The listing builds one solid part. Answer for the finished solid, in the listing's coordinates (mm). A direction names the side the tool comes from. Give positions to 0.01 mm unless a question says otherwise; leave off trailing zeros. Order: outer loops, then holes, each group sorted by start corner. A loop starts at its lowest first (then second) coordinate and runs counter-clockwise, first axis right, second up. Notation, with made-up numbers: (73, 29) - (96, 29) arc R25 cw to (96, 60) - close; hole circle Ø10 at (56, -4). An arc over 180 degrees is marked (long way). Answer in a Markdown table with one row per item.
from build123d import *

# Parameters (mm, degrees)
EXTRUDE1_DEPTH = 3.175
EXTRUDE2_DEPTH = 2.8575


with BuildPart() as part:
    # Sketch1 → Extrude1 (new body)
    with BuildSketch(Plane(origin=(0, 0, 0), x_dir=(1, 0, 0), z_dir=(0, 1, 0))):
        with BuildLine():
            Line((3.175, 44.50785877), (45.047498502, 44.50785877))
            ThreePointArc((45.047498502, 44.50785877), (46.651643951, 44.072811758), (47.81618078, 42.886893339))
            Line((47.81618078, 42.886893339), (87.038547596, -26.992036046))
            ThreePointArc((87.038547596, -26.992036046), (87.009818306, -30.150216064), (84.269865318, -31.721070615))
            Line((84.269865318, -31.721070615), (32.528914715, -31.721070615))
            ThreePointArc((32.528914715, -31.721070615), (30.778624678, -31.195053398), (29.608292243, -29.791297251))
            Line((29.608292243, -29.791297251), (17.72934795, -1.929773364))
            ThreePointArc((17.72934795, -1.929773364), (16.559015516, -0.526017217), (14.808725478, 0))
            Line((14.808725478, 0), (3.175, 0))
            ThreePointArc((3.175, 0), (0.92993597, 0.92993597), (0, 3.175))
            Line((0, 3.175), (0, 41.33285877))
            ThreePointArc((0, 41.33285877), (0.92993597, 43.5779228), (3.175, 44.50785877))
        make_face()
        with BuildLine():
            Line((13.029814646, 30.876332876), (13.029814646, 29.987332876))
            ThreePointArc((13.029814646, 29.987332876), (13.178604401, 29.628122631), (13.537814646, 29.479332876))
            Line((13.537814646, 29.479332876), (15.569814646, 29.479332876))
            ThreePointArc((15.569814646, 29.479332876), (15.929024891, 29.628122631), (16.077814646, 29.987332876))
            Line((16.077814646, 29.987332876), (16.077814646, 30.876332876))
            ThreePointArc((16.077814646, 30.876332876), (16.226604401, 31.235543121), (16.585814646, 31.384332876))
            Line((16.585814646, 31.384332876), (17.474814646, 31.384332876))
            ThreePointArc((17.474814646, 31.384332876), (17.834024891, 31.533122631), (17.982814646, 31.892332876))
            Line((17.982814646, 31.892332876), (17.982814646, 33.924332876))
            ThreePointArc((17.982814646, 33.924332876), (17.834024891, 34.283543121), (17.474814646, 34.432332876))
            Line((17.474814646, 34.432332876), (16.585814646, 34.432332876))
            ThreePointArc((16.585814646, 34.432332876), (16.226604401, 34.581122631), (16.077814646, 34.940332876))
            Line((16.077814646, 34.940332876), (16.077814646, 35.829332876))
            ThreePointArc((16.077814646, 35.829332876), (15.929024891, 36.188543121), (15.569814646, 36.337332876))
            Line((15.569814646, 36.337332876), (13.537814646, 36.337332876))
            ThreePointArc((13.537814646, 36.337332876), (13.178604401, 36.188543121), (13.029814646, 35.829332876))
            Line((13.029814646, 35.829332876), (13.029814646, 34.940332876))
            ThreePointArc((13.029814646, 34.940332876), (12.881024891, 34.581122631), (12.521814646, 34.432332876))
            Line((12.521814646, 34.432332876), (11.632814646, 34.432332876))
            ThreePointArc((11.632814646, 34.432332876), (11.273604401, 34.283543121), (11.124814646, 33.924332876))
            Line((11.124814646, 33.924332876), (11.124814646, 31.892332876))
            ThreePointArc((11.124814646, 31.892332876), (11.273604401, 31.533122631), (11.632814646, 31.384332876))
            Line((11.632814646, 31.384332876), (12.521814646, 31.384332876))
            ThreePointArc((12.521814646, 31.384332876), (12.881024891, 31.235543121), (13.029814646, 30.876332876))
        make_face(mode=Mode.SUBTRACT)
    extrude(amount=-EXTRUDE1_DEPTH)

    # Sketch4 → Extrude2 (add, symmetric)
    with BuildSketch(Plane(origin=(0, 0, 0), x_dir=(1, 0, 0), z_dir=(0, 1, 0))):
        with BuildLine():
            Line((15.569814646, 36.337332876), (13.537814646, 36.337332876))
            ThreePointArc((13.537814646, 36.337332876), (13.178604401, 36.188543121), (13.029814646, 35.829332876))
            Line((13.029814646, 35.829332876), (13.029814646, 34.940332876))
            ThreePointArc((13.029814646, 34.940332876), (12.881024891, 34.581122631), (12.521814646, 34.432332876))
            Line((12.521814646, 34.432332876), (11.632814646, 34.432332876))
            ThreePointArc((11.632814646, 34.432332876), (11.273604401, 34.283543121), (11.124814646, 33.924332876))
            Line((11.124814646, 33.924332876), (11.124814646, 31.892332876))
            ThreePointArc((11.124814646, 31.892332876), (11.273604401, 31.533122631), (11.632814646, 31.384332876))
            Line((11.632814646, 31.384332876), (12.521814646, 31.384332876))
            ThreePointArc((12.521814646, 31.384332876), (12.881024891, 31.235543121), (13.029814646, 30.876332876))
            Line((13.029814646, 30.876332876), (13.029814646, 29.987332876))
            ThreePointArc((13.029814646, 29.987332876), (13.178604401, 29.628122631), (13.537814646, 29.479332876))
            Line((13.537814646, 29.479332876), (15.569814646, 29.479332876))
            ThreePointArc((15.569814646, 29.479332876), (15.929024891, 29.628122631), (16.077814646, 29.987332876))
            Line((16.077814646, 29.987332876), (16.077814646, 30.876332876))
            ThreePointArc((16.077814646, 30.876332876), (16.226604401, 31.235543121), (16.585814646, 31.384332876))
            Line((16.585814646, 31.384332876), (17.474814646, 31.384332876))
            ThreePointArc((17.474814646, 31.384332876), (17.834024891, 31.533122631), (17.982814646, 31.892332876))
            Line((17.982814646, 31.892332876), (17.982814646, 33.924332876))
            ThreePointArc((17.982814646, 33.924332876), (17.834024891, 34.283543121), (17.474814646, 34.432332876))
            Line((17.474814646, 34.432332876), (16.585814646, 34.432332876))
            ThreePointArc((16.585814646, 34.432332876), (16.226604401, 34.581122631), (16.077814646, 34.940332876))
            Line((16.077814646, 34.940332876), (16.077814646, 35.829332876))
            ThreePointArc((16.077814646, 35.829332876), (15.929024891, 36.188543121), (15.569814646, 36.337332876))
        make_face()
    extrude(amount=EXTRUDE2_DEPTH, both=True)


solid = part.part
Item 1: Find section C-C on z = 13. Write down the section's boundary in (x, y) (3 decimals).
Answer block:
| item | result |
|---|---|
| outline | (22.449, -3.175) - (79.185, -3.175) - (79.185, 0) - (22.449, 0) - close |
Item 2: Determine the mould class of faces 4 (the face through (46.631, -1.565, -44.085)), 5 (the face through (11.125, 1, -33)), 6 (the face through (15, -2.858, -33)) for opening direction Z: pulls with the +Z half, pulls with the -Z half, needs draft (parallel to the pull), parting line crosses it, or undercut.
Answer block:
| item | result |
|---|---|
| face 4 | pulls with the -Z half |
| face 5 | needs draft |
| face 6 | undercut |
Item 3: Consider line 1 (Y direction, x = 54, z = -5) (3 decimals); line 2 (Z direction, x = 11, y = -1.25); line 3 (Y direction, x = 13, z = -33.5). Determine where each line is inside the solid, lowest interval first.
Answer block:
| item | result |
|---|---|
| line 1 | -3.175 to 0 |
| line 2 | -44.51 to 0 |
| line 3 | -2.86 to 2.86 |
Item 4: Which of the six approach directions +Z, -Z, +X, -X, +Y, -Y give full straight-line access (tool end or side, diameter ignored) to faces 1 (the face through (17.983, 1, -33)), 2 (the face through (9, -2, 0)), 3 (the face through (15, 1, -36.337))?
Answer block:
| item | result |
|---|---|
| face 1 | +Z, -Z, +X, +Y |
| face 2 | +Z, -X, +Y, -Y |
| face 3 | -Z, +X, -X, +Y |
Item 5: Find section B-B on x = 42.5. Write down the section's boundary in (y, z) (3 decimals).
Answer block:
| item | result |
|---|---|
| outline | (-3.175, -44.508) - (0, -44.508) - (0, 31.721) - (-3.175, 31.721) - close |
Item 6: Each of these flat-tipped pins is pushed along its axis until it touches: P1, Ø4, axis at x = 66.5, z = -14, coming from the +Y side; P2, Ø0.7, axis at x = 12, y = 1.5, coming from the -Z side; P3, Ø6, axis at x = 56.5, z = -28.5, coming from the +Y side; P4, Ø1, axis at y = 1.5, z = -33, coming from the +X side. Where does it stop, or does it pass through?
Answer block:
| item | result |
|---|---|
| P1 | through |
| P2 | z = -34.43 |
| P3 | y = 0 |
| P4 | x = 17.98 |
